Could you check a few things on this model? Use its own coordinates, in mm. A direction names the side the tool comes from. Round coordinates to 2 decimals unless told otherwise and drop trailing zeros. Loops run counter-clockwise (first coordinate to the right, second up) from the corner with the lowest first, then second, coordinate; pieces in that order, holes last. Notation, with made-up numbers: (60.5, 71.5) -> (96.5, 71.5) arc R10 ccw to (96.5, 83.5) -> close; hole circle Ø11 at (-14.75, 86). An arc over 180 degrees is marked (long way). Write each question's results on one line, items separated by ' | '.
from build123d import *

# Parameters (mm, degrees)
BOSS_EXTRUDE1_DEPTH = 5
SKETCH2_R           = 2.5
CUT_EXTRUDE1_DEPTH  = 136.300591277


with BuildPart() as part:
    # Sketch1 → Boss-Extrude1 (new body)
    with BuildSketch(Plane(origin=(0, 0, 0), x_dir=(1, 0, 0), z_dir=(0, 1, 0))):
        with BuildLine():
            Line((-75, 15.75), (-75, -15.75))
            Line((-75, -15.75), (-54, -15.75))
            Line((-54, -15.75), (-54, -79.875))
            Line((-54, -79.875), (-70.25200942, -79.875))
            ThreePointArc((-70.25200942, -79.875), (-72.104159031, -81.120320055), (-71.649789587, -83.305458181))
            ThreePointArc((-71.649789587, -83.305458181), (0, -112.5), (71.649789587, -83.305458181))
            ThreePointArc((71.649789587, -83.305458181), (72.104159031, -81.120320055), (70.25200942, -79.875))
            Line((70.25200942, -79.875), (54, -79.875))
            Line((54, -79.875), (54, -15.75))
            Line((54, -15.75), (75, -15.75))
            Line((75, -15.75), (75, 0))
            Line((75, 0), (75, 15.75))
            Line((75, 15.75), (54, 15.75))
            Line((54, 15.75), (54, 79.875))
            Line((54, 79.875), (70.25200942, 79.875))
            ThreePointArc((70.25200942, 79.875), (72.104159031, 81.120320055), (71.649789587, 83.305458181))
            ThreePointArc((71.649789587, 83.305458181), (0, 112.5), (-71.649789587, 83.305458181))
            ThreePointArc((-71.649789587, 83.305458181), (-72.104159031, 81.120320055), (-70.25200942, 79.875))
            Line((-70.25200942, 79.875), (-54, 79.875))
            Line((-54, 79.875), (-54, 15.75))
            Line((-54, 15.75), (-75, 15.75))
        make_face()
    extrude(amount=BOSS_EXTRUDE1_DEPTH)

    # Sketch2 → Cut-Extrude1 (cut, through all)
    with BuildSketch(Plane(origin=(0, 5, 0), x_dir=(1, 0, 0), z_dir=(0, 1, 0))):
        with Locations(Location((-62.5, 85, 0), (0, 0, 270))):
            Circle(SKETCH2_R)
        with Locations(Location((62.5, 85, 0), (0, 0, 270))):
            Circle(SKETCH2_R)
        with Locations(Location((62.5, 0, 0), (0, 0, 270))):
            Circle(SKETCH2_R)
        with Locations(Location((62.5, -85, 0), (0, 0, 270))):
            Circle(SKETCH2_R)
        with Locations(Location((-62.5, 0, 0), (0, 0, 270))):
            Circle(SKETCH2_R)
        with Locations(Location((-62.5, -85, 0), (0, 0, 270))):
            Circle(SKETCH2_R)
    extrude(amount=-CUT_EXTRUDE1_DEPTH, mode=Mode.SUBTRACT)


solid = part.part
1) I want a section at D-D, the plane z = 60.5. Write out the boundary of the cut face in (x, y), plus the area to 3 significant figures.
Model answer:
outline: (-54, 0) -> (54, 0) -> (54, 5) -> (-54, 5) -> close | area: 540 mm2
2) I want a section at B-B, the plane z = 0. Write out the boundary of the cut face in (x, y), plus the area to 3 significant figures.
Model answer:
outline: (-75, 0) -> (-65, 0) -> (-65, 5) -> (-75, 5) -> close; (-60, 0) -> (60, 0) -> (60, 5) -> (-60, 5) -> close; (65, 0) -> (75, 0) -> (75, 5) -> (65, 5) -> close | area: 700 mm2
3) For faces 1 (the flat face through (-62, 2, 79.875)), 2 (the flat face through (54, 2, 48)), 3 (the cylindrical face through (-1.111, 2.465, 112.494)), which set-ups out of +Z, -Z, +X, -X, +Y, -Y let a thin tool reach every point of the face, with its end or its side?
Model answer:
face 1: -X, +Y, -Y | face 2: +X, +Y, -Y | face 3: +Z, +Y, -Y
4) I'm going to push flat-ended pins straight in: pin 1 (1 mm diameter, centred on y = 4.5, z = -85.5, fed in from +X); pin 2 (4 mm diameter, centred on x = 62.5, z = -85, fed in from -Y); pin 3 (2 mm diameter, centred on y = 2, z = 32.5, fed in from -X); pin 4 (2.5 mm diameter, centred on x = -63, y = 2, fed in from +Z). Where does each tip first touch, or does it pass through?
Model answer:
pin 1: stops at x = 69.87 | pin 2: passes through | pin 3: stops at x = -54 | pin 4: stops at z = 91.82
5) I need wall thicknesses on line 1 (X direction, y = 2.3, z = 0); line 2 (Z direction, x = 64, y = 2.15) (3 decimals); line 3 (X direction, y = 3.55, z = -85). Which ranges of each line are inside material? Lowest first, please.
Model answer:
line 1: x = -75 to -65, -60 to 60, 65 to 75 | line 2: z = -90.069 to -87, -83 to -79.875, -15.75 to -2, 2 to 15.75, 79.875 to 83, 87 to 90.069 | line 3: x = -69.87 to -65, -60 to 60, 65 to 69.87
6) I want a section at C-C, the plane x = -62.5. Write out the boundary of the cut face in (y, z) (3 decimals).
Model answer:
outline: (0, -91.245) -> (5, -91.245) -> (5, -87.5) -> (0, -87.5) -> close; (0, -82.5) -> (5, -82.5) -> (5, -79.875) -> (0, -79.875) -> close; (0, -15.75) -> (5, -15.75) -> (5, -2.5) -> (0, -2.5) -> close; (0, 2.5) -> (5, 2.5) -> (5, 15.75) -> (0, 15.75) -> close; (0, 79.875) -> (5, 79.875) -> (5, 82.5) -> (0, 82.5) -> close; (0, 87.5) -> (5, 87.5) -> (5, 91.245) -> (0, 91.245) -> close
7) I want a section at A-A, the plane y = 3.4. Write out the boundary of the cut face in (x, z) (3 decimals), plus the area to 3 significant figures.
Model answer:
outline: (-75, -15.75) -> (-54, -15.75) -> (-54, -79.875) -> (-70.252, -79.875) arc R2 ccw to (-71.65, -83.305) arc R102.519 ccw to (71.65, -83.305) arc R2 ccw to (70.252, -79.875) -> (54, -79.875) -> (54, -15.75) -> (75, -15.75) -> (75, 15.75) -> (54, 15.75) -> (54, 79.875) -> (70.252, 79.875) arc R2 ccw to (71.65, 83.305) arc R102.519 ccw to (-71.65, 83.305) arc R2 ccw to (-70.252, 79.875) -> (-54, 79.875) -> (-54, 15.75) -> (-75, 15.75) -> close; hole circle Ø5 at (-62.5, -85); hole circle Ø5 at (-62.5, 0); hole circle Ø5 at (-62.5, 85); hole circle Ø5 at (62.5, -85); hole circle Ø5 at (62.5, 0); hole circle Ø5 at (62.5, 85) | area: 25,200 mm2
8) If we mould it in two halves opening along Z, with no side actions, what happens to faces 4 (the cylindrical face through (1.111, 2.465, -112.494)), 5 (the flat face through (-1, 5, -2)), 6 (the flat face through (-65, 2, 15.75))? For each: released by +Z, released by -Z, zero draft, split by the parting line, or undercut.
Model answer:
face 4: released by -Z | face 5: zero draft | face 6: undercut
